Job drawing, mm, ordinate dimensions from the low corner. One solid piece. Coordinates: 2 decimals unless noted, no trailing zeros. Order: outer loops, then holes, each group sorted by start corner. A loop starts at its lowest first (then second) coordinate and runs counter-clockwise, first axis right, second up. Notation, with made-up numbers: (-23.75, 59.5) - (9.25, 59.5) arc R11 ccw to (9.25, 72.5) - close; hole circle Ø9 at (38.25, 57). An arc over 180 degrees is marked (long way). Return JSON: item names as keys, results as strings.
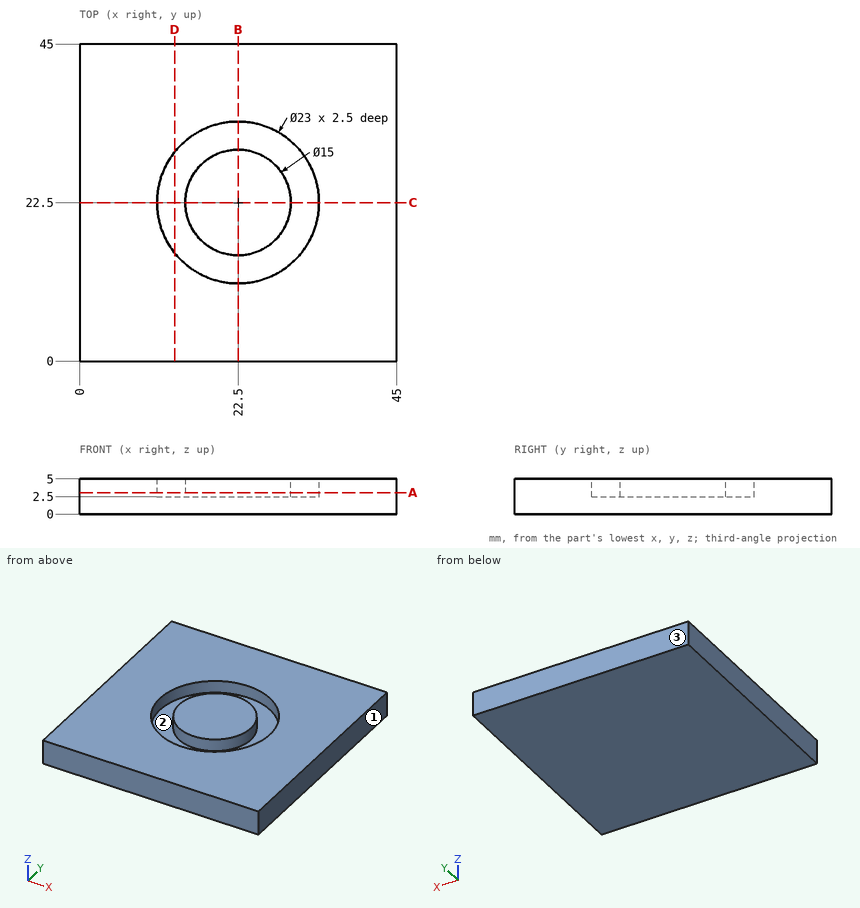
1. Cut at A-A on z = 3.05. Give the cut face in (x, y), plus the area to 3 significant figures.
Check values:
{"outline": "(0, 0) - (45, 0) - (45, 45) - (0, 45) - close; circle Ø15 at (22.5, 22.5); hole circle Ø23 at (22.5, 22.5)", "area": "1,790 mm²"}
2. Mould opens along X. For the marked faces 1, 2 and 3 say: pulls with the +X half, pulls with the -X half, needs draft (parallel to the pull), parting line crosses it, or undercut.
Check values:
{"face 1": "pulls with the +X half", "face 2": "undercut", "face 3": "needs draft"}
3. Cut at B-B on x = 22.5. Give the cut face in (y, z).
Check values:
{"outline": "(0, 0) - (45, 0) - (45, 5) - (34, 5) - (34, 2.5) - (30, 2.5) - (30, 5) - (15, 5) - (15, 2.5) - (11, 2.5) - (11, 5) - (0, 5) - close"}
4. Probe L1, parallel to Y at x = 22.5, z = 3.7; L2, parallel to Y at x = 21, z = 3.9. List the from-to ranges inside material, lowest first.
Check values:
{"L1": "0 to 11, 15 to 30, 34 to 45", "L2": "0 to 11.1, 15.15 to 29.85, 33.9 to 45"}
5. Cut at D-D on x = 13.5. Give the cut face in (y, z), plus the area to 3 significant figures.
Check values:
{"outline": "(0, 0) - (45, 0) - (45, 5) - (29.66, 5) - (29.66, 2.5) - (15.34, 2.5) - (15.34, 5) - (0, 5) - close", "area": "189 mm²"}
